```python
from build123d import *

# Parameters (mm, degrees)
SKETCH1_W           = 42
SKETCH1_H           = 42
SKETCH1_R           = 1.55
BOSS_EXTRUDE1_DEPTH = 25
SKETCH2_R           = 1.65
SKETCH2_R_2         = 11
CUT_EXTRUDE1_DEPTH  = 25
SKETCH3_R           = 2.9
CUT_EXTRUDE2_DEPTH  = 3
CHAMFER1_SIZE       = 2
SKETCH4_R           = 18.15
CUT_EXTRUDE3_DEPTH  = 18.5
CUT_EXTRUDE_1_DEPTH = 4


with BuildPart() as part:
    # Sketch1 → Boss-Extrude1 (new body)
    with BuildSketch(Plane.XY):
        Rectangle(SKETCH1_W, SKETCH1_H)
        with Locations((-15.5, 15.5)):
            Circle(SKETCH1_R, mode=Mode.SUBTRACT)
        with Locations((15.5, 15.5)):
            Circle(SKETCH1_R, mode=Mode.SUBTRACT)
        with Locations((15.5, -15.5)):
            Circle(SKETCH1_R, mode=Mode.SUBTRACT)
        with Locations((-15.5, -15.5)):
            Circle(SKETCH1_R, mode=Mode.SUBTRACT)
    extrude(amount=BOSS_EXTRUDE1_DEPTH)

    # Sketch2 → Cut-Extrude1 (cut)
    with BuildSketch(Plane.XY.offset(25)):
        with Locations((9.899494937, 9.899494937)):
            Circle(SKETCH2_R)
        with Locations((9.899494937, -9.899494937)):
            Circle(SKETCH2_R)
        with Locations((-9.899494937, -9.899494937)):
            Circle(SKETCH2_R)
        with Locations((-9.899494937, 9.899494937)):
            Circle(SKETCH2_R)
        Circle(SKETCH2_R_2)
    extrude(amount=-CUT_EXTRUDE1_DEPTH, mode=Mode.SUBTRACT)

    # Sketch3 → Cut-Extrude2 (cut)
    with BuildSketch(Plane.XY.offset(25)):
        with Locations((9.899494937, 9.899494937)):
            Circle(SKETCH3_R)
        with Locations((9.899494937, -9.899494937)):
            Circle(SKETCH3_R)
        with Locations((-9.899494937, -9.899494937)):
            Circle(SKETCH3_R)
        with Locations((-9.899494937, 9.899494937)):
            Circle(SKETCH3_R)
    extrude(amount=-CUT_EXTRUDE2_DEPTH, mode=Mode.SUBTRACT)

    # Chamfer1
    chamfer1_edges = [part.edges().sort_by_distance(p)[0] for p in [
        (21, -21, 12.5),
        (-21, -21, 12.5),
        (-21, 21, 12.5),
        (21, 21, 12.5),
    ]]
    chamfer(chamfer1_edges, length=CHAMFER1_SIZE)

    # Sketch4 → Cut-Extrude3 (cut)
    with BuildSketch(Plane(origin=(0, 0, 0), x_dir=(-1, 0, 0), z_dir=(0, 0, -1))):
        Circle(SKETCH4_R)
    extrude(amount=-CUT_EXTRUDE3_DEPTH, mode=Mode.SUBTRACT)

    # 草图1 → 切除-拉伸1 (cut)
    with BuildSketch(Plane.XY):
        Polygon((-15.5, 12.209103466), (-12.65, 13.854551733), (-12.65, 17.145448267), (-15.5, 18.790896534), (-18.35, 17.145448267), (-18.35, 13.854551733), align=None)
        Polygon((15.5, -12.209103466), (12.65, -13.854551733), (12.65, -17.145448267), (15.5, -18.790896534), (18.35, -17.145448267), (18.35, -13.854551733), align=None)
        Polygon((15.5, 18.790896534), (12.65, 17.145448267), (12.65, 13.854551733), (15.5, 12.209103466), (18.35, 13.854551733), (18.35, 17.145448267), align=None)
        Polygon((-15.5, -12.209103466), (-18.35, -13.854551733), (-18.35, -17.145448267), (-15.5, -18.790896534), (-12.65, -17.145448267), (-12.65, -13.854551733), align=None)
    extrude(amount=CUT_EXTRUDE_1_DEPTH, mode=Mode.SUBTRACT)


solid = part.part
```
Can you work these out from the model? Positions are in its coordinate system, mm. A direction names the side the tool comes from. Coordinates: 2 decimals unless noted, no trailing zeros. Order: outer loops, then holes, each group sorted by start corner. A loop starts at its lowest first (then second) coordinate and runs counter-clockwise, first axis right, second up.
1. If we section it at B-B (z = 16): Please give me the cut outline in (x, y).
2. For faces 1 (the face through (16.94, -13.04, 1.97)), 2 (the face through (8.683, -8.784, 20.274)), 3 (the face through (12, 10, 22)), which set-ups out of +Z, -Z, +X, -X, +Y, -Y let a thin tool reach every point of the face, with its end or its side?
3. I'm going to push flat-ended pins straight in: pin 1 (4.5 mm diameter, centred on x = -9.9, y = -9.9, fed in from -Z); pin 2 (3.5 mm diameter, centred on x = -9.9, y = -9.9, fed in from +Z); pin 3 (1.5 mm diameter, centred on x = -15, y = -10, fed in from -Z); pin 4 (3 mm diameter, centred on x = -16, y = 16.5, fed in from -Z). Where does each tip first touch, or does it pass through?
4. I need wall thicknesses on line 1 (Y direction, x = 0, z = 13.5); line 2 (Y direction, x = -16.5, z = 10.5); line 3 (Y direction, x = 16, z = 11.5). Which ranges of each line are inside material? Lowest first, please.
5. If we section it at A-A (y = 0): Please give me the cut outline in (x, z).
6. Thinking about a two-plate mould opening in Y: for faces 4 (the face through (-18.35, -15, 2)), 5 (the face through (20, -20, 12)), 6 (the face through (-20, 20, 12)), 7 (the face through (-8, -8, 18.5)), which applies, +Y half, -Y half, draft (parallel to the pull), parting line (faces both ways), or undercut?
7. If we section it at D-D (x = 16.5): Please give me the cut outline in (y, z), then the cut area to 3 significant figures.
Entries:
1. outline: (-21, -19) - (-19, -21) - (19, -21) - (21, -19) - (21, 19) - (19, 21) - (-19, 21) - (-21, 19) - close; hole circle Ø36.3 at (0, 0); hole circle Ø3.1 at (-15.5, -15.5); hole circle Ø3.1 at (-15.5, 15.5); hole circle Ø3.1 at (15.5, -15.5); hole circle Ø3.1 at (15.5, 15.5)
2. face 1: -Z
2. face 2: +Z, -Z
2. face 3: +Z
3. pin 1: stops at z = 18.5
3. pin 2: stops at z = 22
3. pin 3: stops at z = 0
3. pin 4: stops at z = 4
4. line 1: y = -21 to -18.15, 18.15 to 21
4. line 2: y = -21 to -16.68, -14.32 to -7.56, 7.56 to 14.32, 16.68 to 21
4. line 3: y = -21 to -16.97, -14.03 to -8.57, 8.57 to 14.03, 16.97 to 21
5. outline: (-21, 0) - (-18.15, 0) - (-18.15, 18.5) - (-11, 18.5) - (-11, 25) - (-21, 25) - close; (11, 18.5) - (18.15, 18.5) - (18.15, 0) - (21, 0) - (21, 25) - (11, 25) - close
6. face 4: undercut
6. face 5: -Y half
6. face 6: +Y half
6. face 7: undercut
7. outline: (-21, 0) - (-18.21, 0) - (-18.21, 4) - (-16.68, 4) - (-16.68, 25) - (-21, 25) - close; (-14.32, 4) - (-12.79, 4) - (-12.79, 0) - (-7.56, 0) - (-7.56, 18.5) - (7.56, 18.5) - (7.56, 0) - (12.79, 0) - (12.79, 4) - (14.32, 4) - (14.32, 25) - (-14.32, 25) - close; (16.68, 4) - (18.21, 4) - (18.21, 0) - (21, 0) - (21, 25) - (16.68, 25) - close
7. area: 627 mm2
